Build history of the part. All positions in model axes, mm. A direction names the side the tool comes from. Round coordinates to 2 decimals unless told otherwise and drop trailing zeros. Write each loop counter-clockwise with the first axis right and the second up, starting at its lowest first coordinate (ties: lowest second). Pieces come first, ordered by that corner, then holes. Notation, with made-up numbers: (-20, 89.25) -> (4, 89.25) arc R25 cw to (4, 122.25) -> close; hole circle Ø4 at (1, -8.5). An arc over 180 degrees is marked (long way). Answer in a Markdown table with one row per item.
```python
from build123d import *

# Parameters (mm, degrees)
EXTRUDE_4_DEPTH = 150
SKETCH_1_5_R    = 22.5
EXTRUDE_5_DEPTH = 100
EXTRUDE_6_DEPTH = 50
SHELL_START     = 1.5
SHELL_3_DEPTH   = 197
SHELL_3_2_DEPTH = 97


# Read off the part's stored shape, not the designer's step: 抽壳3
with BuildPart() as part:
    # 草图1 → 凸台-拉伸4 (new body)
    with BuildSketch(Plane.XY):
        with BuildLine():
            ThreePointArc((22.5, 0), (11.711646096, 19.211646096), (-10.307764064, 20))
            Line((-10.307764064, 20), (-10.307764064, -20))
            ThreePointArc((-10.307764064, -20), (11.711646096, -19.211646096), (22.5, 0))
        make_face()
    extrude(amount=EXTRUDE_4_DEPTH)

    # 草图1<5> → 凸台-拉伸5 (add)
    with BuildSketch(Plane.XY):
        with Locations(Location((0, 0, 0), (0, 0, 117.266044451))):
            Circle(SKETCH_1_5_R)
    extrude(amount=EXTRUDE_5_DEPTH)

    # 草图4 → 凸台-拉伸6 (add)
    with BuildSketch(Plane.XY.offset(150)):
        with BuildLine():
            ThreePointArc((-10.307764064, -20), (22.5, 0), (-10.307764064, 20))
            Line((-10.307764064, 20), (-10.307764064, -20))
        make_face()
    extrude(amount=EXTRUDE_6_DEPTH)

    # 抽壳3 outline → 抽壳3 (cut)
    with BuildSketch(Plane.XY.offset(SHELL_START)):
        with BuildLine():
            Line((-8.807764064, 19.063664186), (-8.807764064, -19.063664186))
            ThreePointArc((-8.807764064, -19.063664186), (21, 0), (-8.807764064, 19.063664186))
        make_face()
    extrude(amount=SHELL_3_DEPTH, mode=Mode.SUBTRACT)

    # Shell 3 2 outline → Shell 3 2 (cut)
    with BuildSketch(Plane.XY.offset(SHELL_START)):
        with BuildLine():
            ThreePointArc((-8.807764064, 19.063664186), (-21, 0), (-8.807764064, -19.063664186))
            Line((-8.807764064, -19.063664186), (-8.807764064, 19.063664186))
        make_face()
    extrude(amount=SHELL_3_2_DEPTH, mode=Mode.SUBTRACT)


solid = part.part
```
Q1. Saw through at A-A on x = 0. Write the cut outline in (y, z), plus the area to 3 significant figures.
A:
| item | result |
|---|---|
| outline | (-22.5, 0) -> (22.5, 0) -> (22.5, 200) -> (-22.5, 200) -> close; hole (-21, 1.5) -> (21, 1.5) -> (21, 198.5) -> (-21, 198.5) -> close |
| area | 726 mm² |
Q2. Wall check: line 1 (Z direction, x = 17.5, y = 6.5); line 2 (Y direction, x = 0, z = 69.5); line 3 (Z direction, x = -10, y = 15). Give the ranges that are in metal, low to high. Write a range as [from, to].
A:
| item | result |
|---|---|
| line 1 | [0, 1.5], [198.5, 200] |
| line 2 | [-22.5, -21], [21, 22.5] |
| line 3 | [0, 1.5], [98.5, 200] |
Q3. Saw through at D-D on z = 170.5. Write the cut outline in (x, y).
A:
| item | result |
|---|---|
| outline | (-10.31, -20) arc R22.5 ccw (long way) to (-10.31, 20) -> close; hole (-8.81, -19.06) arc R21 ccw (long way) to (-8.81, 19.06) -> close |
Q4. Which spindle directions (+Z, -Z, +X, -X, +Y, -Y) get a long thin tool onto all of the face, cutting with end or side? Do faces 3 (the flat face through (-10.308, 0, 149)), 4 (the flat face through (2, 0, 200)), 5 (the flat face through (3, 0, 198.5)). Say none if no direction does.
A:
| item | result |
|---|---|
| face 3 | +Z, -X, +Y, -Y |
| face 4 | +Z, +X, -X, +Y, -Y |
| face 5 | none |
Q5. Saw through at C-C on y = -17. Write the cut outline in (x, z), plus the area to 3 significant figures.
A:
| item | result |
|---|---|
| outline | (-14.74, 0) -> (14.74, 0) -> (14.74, 200) -> (-10.31, 200) -> (-10.31, 100) -> (-14.74, 100) -> close; hole (-12.33, 1.5) -> (12.33, 1.5) -> (12.33, 198.5) -> (-8.81, 198.5) -> (-8.81, 98.5) -> (-12.33, 98.5) -> close |
| area | 947 mm² |
Q6. Two-plate mould, pull along Y, no slides. Class faces 1 (the flat face through (0, 0, 0)), 2 (the flat face through (-8.808, 0, 148)): released by +Y, released by -Y, zero draft, split by the parting line, or undercut.
A:
| item | result |
|---|---|
| face 1 | zero draft |
| face 2 | undercut |
Q7. Drop flat-ended pins along their axis: P1, Ø1.5, axis at x = 14, z = 91.5, coming from the -Y side; P2, Ø12, axis at x = -8, z = 45.5, coming from the -Y side; P3, Ø10, axis at x = 9.5, y = 10, coming from the -Z side; P4, Ø10, axis at y = 1.5, z = 113.5, coming from the -X side. Give the stop position or say it passes through.
A:
| item | result |
|---|---|
| P1 | y = -18.18 |
| P2 | y = -22.41 |
| P3 | z = 0 |
| P4 | x = -10.31 |
Q8. Saw through at B-B on z = 28.5. Write the cut outline in (x, y), plus the area to 3 significant figures.
A:
| item | result |
|---|---|
| outline | circle Ø45 at (0, 0); hole circle Ø42 at (0, 0) |
| area | 205 mm² |
